CAD build for the part. Positions are in the model's coordinates, mm. Face numbers are marked on the shaded views. A direction names the side the tool comes from. Coordinates: 2 decimals unless noted, no trailing zeros. Loops run counter-clockwise (first coordinate to the right, second up) from the corner with the lowest first, then second, coordinate; pieces in that order, holes last. Notation, with made-up numbers: (77, 10) -> (130, 10) arc R18 cw to (130, 15) -> close; hole circle Ø9 at (-29.5, -36). An arc over 180 degrees is marked (long way). Return JSON: item names as keys, results as strings. Group by question number.
(1) Flat gauge pins, fed straight in: pin 1 Ø2 at (y, z) = (-19, 2) entering from +X; pin 2 Ø2 at (y, z) = (0.5, -4) entering from -X; pin 3 Ø8 at (x, y) = (-56, 2) entering from -Z. Where does each tip first touch, or does it go through?
(2) Saw through at A-A on z = -9.5. Write the cut outline in (x, y), then the cut area to 3 significant figures.
(3) Saw through at D-D on z = -4. Write the cut outline in (x, y), then the cut area to 3 significant figures.
(4) Saw through at C-C on y = 3. Write the cut outline in (x, z), then the cut area to 3 significant figures.
(5) Mould opens along Y. For the marked faces 1, 2 and 3 say: pulls with the +Y half, pulls with the -Y half, needs draft (parallel to the pull), parting line crosses it, or undercut.
(6) Saw through at B-B on x = -38. Write the cut outline in (y, z), then the cut area to 3 significant figures.
(7) Tool access for the marked faces 4, 5, 6, 7 and 8: list every direction of +Z, -Z, +X, -X, +Y, -Y with a clear straight run to the whole face (end or side of a thin tool).
(8) Probe L1, parallel to Y at x = -21, z = -3.5; L2, parallel to Z at x = 2.5, y = -8. List the from-to ranges inside material, lowest first.
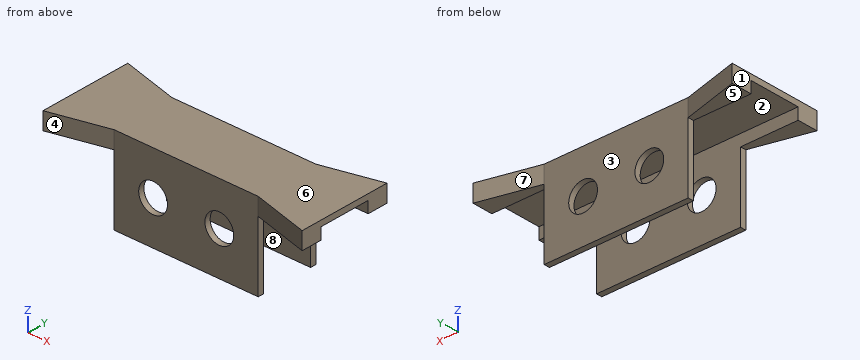
```python
from build123d import *

# Parameters (mm, degrees)
SKETCH1_W           = 50
SKETCH1_H           = 30
SKETCH1_R           = 5
BOSS_EXTRUDE2_DEPTH = 2
BOSS_EXTRUDE3_DEPTH = 2
BOSS_EXTRUDE4_DEPTH = 6


with BuildPart() as part:
    # Sketch1 → Boss-Extrude2 (new body)
    with BuildSketch(Plane(origin=(0, 0, 0), x_dir=(1, 0, 0), z_dir=(0, 1, 0))):
        with Locations((-18.81443299, 0.927835052)):
            Rectangle(SKETCH1_W, SKETCH1_H)
        with Locations(Location((-30.31443299, 0.927835052, 0), (0, 0, 270))):
            Circle(SKETCH1_R, mode=Mode.SUBTRACT)
        with Locations(Location((-7.31443299, 0.927835052, 0), (0, 0, 270))):
            Circle(SKETCH1_R, mode=Mode.SUBTRACT)
    extrude(amount=BOSS_EXTRUDE2_DEPTH)

    # Sketch2 → Boss-Extrude3 (add)
    with BuildSketch(Plane.XY.offset(14.072164948)):
        Polygon((26.18556701, 0), (26.18556701, -9), (-63.81443299, -9), (-63.81443299, 0), (-43.81443299, 0), (6.18556701, 0), align=None)
    extrude(amount=-BOSS_EXTRUDE3_DEPTH)

    # Sketch2_4 → Boss-Extrude4 (add)
    with BuildSketch(Plane.XY.offset(14.072164948)):
        Polygon((26.18556701, 7.203034525), (26.18556701, 0), (6.18556701, 0), (6.18556701, 2), align=None)
        Polygon((-43.81443299, 2), (-63.81443299, 7.203034525), (-63.81443299, 0), (-43.81443299, 0), align=None)
    extrude(amount=-BOSS_EXTRUDE4_DEPTH)

    # Mirror1: part across plane


with BuildPart() as part_1:
    add(part.part)
    add(part.part.mirror(Plane(origin=(0, -9, 12.072164948), x_dir=(0, 0, 1), z_dir=(0, -1, 0))))


solid = part_1.part
```
Geometry results:
{
 "1": {"pin 1": "x = 6.19", "pin 2": "x = -43.81", "pin 3": "z = 8.07"},
 "2": {"outline": "(-43.81, -20) -> (6.19, -20) -> (6.19, -18) -> (-43.81, -18) -> close; (-43.81, 0) -> (6.19, 0) -> (6.19, 2) -> (-43.81, 2) -> close", "area": "200 mm²"},
 "3": {"outline": "(-43.81, -20) -> (-34.26, -20) -> (-34.26, -18) -> (-43.81, -18) -> close; (-43.81, 0) -> (-34.26, 0) -> (-34.26, 2) -> (-43.81, 2) -> close; (-26.37, -20) -> (-11.26, -20) -> (-11.26, -18) -> (-26.37, -18) -> close; (-26.37, 0) -> (-11.26, 0) -> (-11.26, 2) -> (-26.37, 2) -> close; (-3.37, -20) -> (6.19, -20) -> (6.19, -18) -> (-3.37, -18) -> close; (-3.37, 0) -> (6.19, 0) -> (6.19, 2) -> (-3.37, 2) -> close", "area": "137 mm²"},
 "4": {"outline": "(-63.81, 8.07) -> (-47.66, 8.07) -> (-47.66, 14.07) -> (-63.81, 14.07) -> close; (10.03, 8.07) -> (26.19, 8.07) -> (26.19, 14.07) -> (10.03, 14.07) -> close", "area": "194 mm²"},
 "5": {"face 1": "needs draft", "face 2": "undercut", "face 3": "pulls with the +Y half"},
 "6": {"outline": "(-20, -15.93) -> (-18, -15.93) -> (-18, 12.07) -> (0, 12.07) -> (0, -15.93) -> (2, -15.93) -> (2, 14.07) -> (-20, 14.07) -> close", "area": "156 mm²"},
 "7": {"face 4": "+Z, -Z, -Y", "face 5": "-Z, -X, +Y, -Y", "face 6": "+Z, +X, -X, +Y, -Y", "face 7": "+Z, -Z, +Y", "face 8": "-Z, +X, -X"},
 "8": {"L1": "-20 to -18, 0 to 2", "L2": "12.07 to 14.07"}
}
